Source: CAD feature listing. Evaluate the final solid. Frame: model axes, mm. Face numbers are marked on the shaded views. Give positions to 0.01 mm unless a question says otherwise; leave off trailing zeros. Order: outer loops, then holes, each group sorted by start corner. A loop starts at its lowest first (then second) coordinate and runs counter-clockwise, first axis right, second up. Notation, with made-up numbers: (9.5, 33.25) -> (22.5, 33.25) arc R35 ccw to (22.5, 69.25) -> close; hole circle Ø5 at (50.5, 68). An arc over 180 degrees is marked (long way). Use CSV: the item, a comma, the result in double quotes.
Autodesk Inventor part; units mm, degrees
ref_plane "YZ Plane" through (0, 0, 0) normal (1, 0, 0) x (0, 1, 0)
ref_plane "XZ Plane" through (0, 0, 0) normal (0, 1, 0) x (-1, 0, 0)
ref_plane "XY Plane" through (0, 0, 0) normal (0, 0, 1) x (1, 0, 0)
sketch "Sketch1" plane through (0, 0, 0) normal (0, 1, 0) x (-1, 0, 0)
  line L0 (6.29, 17.6429) -> (-24.19, 17.6429)
  line L1 (-24.19, 17.6429) -> (-24.19, -14.3571)
  line L2 (-24.19, -14.3571) -> (6.29, -14.3571)
  line L3 (6.29, -14.3571) -> (6.29, 17.6429)
  point P0 (0, 0)
  dimension "d0" = 30.48
  dimension "d1" = 32
extrude "Extrusion1" add sketch "Sketch1" along normal blind 2
sketch "Sketch3" plane through (0, 2, 0) normal (0, 1, 0) x (1, 0, 0)
  line L0 (-6.29, -17.6429) -> (24.19, -17.6429)
  line L1 (-6.29, -17.6429) -> (-6.29, -16.6429)
  line L2 (-6.29, 14.3571) -> (-6.29, -17.6429)
  line L3 (-6.29, -16.6429) -> (-5.29, -16.6429)
  line L4 (-5.29, -16.6429) -> (-5.29, 13.3571)
  line L5 (24.19, 14.3571) -> (-6.29, 14.3571)
  line L6 (24.19, -17.6429) -> (24.19, 14.3571)
  line L7 (24.19, -17.6429) -> (23.19, -17.6429)
  line L8 (23.19, -17.6429) -> (23.19, -16.6429)
  line L9 (23.19, -16.6429) -> (23.19, 3.3571)
  line L10 (23.19, -16.6429) -> (-5.29, -16.6429)
  line L11 (-5.29, -16.6429) -> (-5.29, 13.3571)
  line L12 (-5.29, 13.3571) -> (23.19, 13.3571)
  line L13 (23.19, 13.3571) -> (23.19, -16.6429)
  point P0 (0, 0)
  dimension "d4" = 1
  dimension "d5" = 1
  dimension "d6" = 30
  dimension "d7" = 1
extrude "Extrusion3" add sketch "Sketch3" along normal blind 1 contours L1 L3 L10 L8 L0 | L8 L9 L13 L12 L4 L3 L2 L5 L6 L0
sketch "Sketch4" plane through (0, 0, 0) normal (0, -1, 0) x (1, 0, 0)
  line L0 (24.19, -14.3571) -> (-6.29, -14.3571)
  line L1 (8.95, -14.3571) -> (8.95, -7.3571)
  point P0 (0, 0)
  dimension "d12" = 7
hole "Hole1" at (8.95, 0, -7.3571) direction (0, 1, 0) diameter 9 end through all
sketch "Sketch5" plane through (0, 3, 0) normal (0, 1, 0) x (1, 0, 0)
  line L0 (-6.29, -17.6429) -> (24.19, -17.6429)
  line L1 (8.95, -17.6429) -> (8.95, -0.6429)
  line L2 (8.95, -0.6429) -> (24.19, -0.6429)
  line L3 (24.19, -17.6429) -> (24.19, 14.3571)
  line L4 (24.19, -0.6429) -> (24.19, -4.1429)
  line L5 (24.19, -4.1429) -> (23.19, -4.1429)
  line L6 (23.19, -16.6429) -> (23.19, 13.3571)
  line L7 (23.19, -4.1429) -> (23.19, 2.8571)
  line L8 (23.19, 2.8571) -> (24.19, 2.8571)
  line L9 (24.19, 2.8571) -> (24.19, -4.1429)
  line L10 (-5.29, -16.6429) -> (-5.29, 13.3571)
  line L11 (-5.29, -0.6429) -> (-5.29, -4.1429)
  line L12 (-5.29, -4.1429) -> (-6.29, -4.1429)
  line L13 (-6.29, 14.3571) -> (-6.29, -17.6429)
  line L14 (-6.29, -4.1429) -> (-6.29, 2.8571)
  line L15 (-6.29, 2.8571) -> (-5.29, 2.8571)
  line L16 (-5.29, -0.6429) -> (-5.29, 2.8571)
  point P0 (0, 0)
  dimension "d20" = 17
  dimension "d21" = 3.5
  dimension "d22" = 7
  dimension "d23" = 7
sketch "Sketch6" plane through (0, 0, 0) normal (0, -1, 0) x (1, 0, 0)
  line L0 (-5.29, 4.1429) -> (-6.29, 4.1429)
  line L1 (-6.29, -2.8571) -> (-5.29, -2.8571)
  line L2 (23.19, -2.8571) -> (24.19, -2.8571)
  line L3 (24.19, 4.1429) -> (23.19, 4.1429)
  line L4 (-5.29, -13.3571) -> (-5.29, 16.6429)
  line L5 (-6.29, -14.3571) -> (-6.29, 17.6429)
  line L6 (23.19, 16.6429) -> (23.19, -13.3571)
  line L7 (24.19, 17.6429) -> (24.19, -14.3571)
  line L8 (24.19, 4.1429) -> (29.19, 4.1429)
  line L9 (29.19, 4.1429) -> (29.19, -2.8571)
  line L10 (29.19, -2.8571) -> (24.19, -2.8571)
  line L11 (-6.29, -2.8571) -> (-11.29, -2.8571)
  line L12 (-11.29, -2.8571) -> (-11.29, 4.1429)
  line L13 (-11.29, 4.1429) -> (-6.29, 4.1429)
  point P0 (0, 0)
  dimension "d26" = 5
  dimension "d27" = 5
extrude "Extrusion5" add sketch "Sketch6" against normal blind 3 contours L5 L11 L12 L13 | L7 L8 L9 L10
sketch "Sketch7" plane through (0, 0, 0) normal (0, -1, 0) x (1, 0, 0)
  line L0 (-6.29, 17.6429) -> (24.19, 17.6429)
  line L1 (8.95, 17.6429) -> (8.95, 0.6429)
  line L2 (8.95, 0.6429) -> (26.45, 0.6429)
  line L3 (26.45, 0.6429) -> (-8.55, 0.6429)
  point P0 (0, 0)
  dimension "d30" = 17
  dimension "d31" = 17.5
  dimension "d32" = 35
hole "Hole2" at (-8.55, 0, 0.6429) at (26.45, 0, 0.6429) direction (0, 1, 0) diameter 4 end through all
sketch "Sketch8" plane through (-6.29, 0, 17.6429) normal (0, 0, 1) x (1, 0, 0)
  line L0 (0, 0) -> (0, 3)
  line L1 (1, 3) -> (0, 3)
  line L2 (1, 3) -> (1, 3.5)
  line L3 (0, 3.5) -> (1, 3.5)
  line L4 (-5, 0) -> (-5, 3.25)
  line L5 (0, 0) -> (-5, 0)
  line L6 (0, 3) -> (0, 0)
  line L7 (0, 0) -> (30.48, 0)
  line L8 (30.48, 0) -> (30.48, 3)
  line L9 (0, 3) -> (30.48, 3)
  line L10 (0, 0) -> (0, 3)
  line L11 (0, 3.25) -> (0, 3.5)
  line L12 (-5, 3.25) -> (0, 3.25)
  point P0 (6.29, 0)
extrude "Extrusion6" cut sketch "Sketch8" against normal blind 0.2 contours L0 L1 L9 L8 L7
properties part number "sheel"
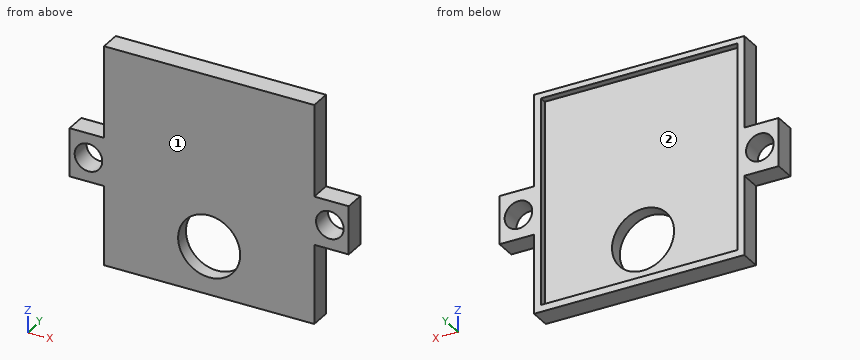
1. Mould query, pull axis Z, two halves, no side actions, for the marked faces 1 and 2. Classes: released by +Z, released by -Z, zero draft, split by the parting line, or undercut.
Answer below:
face 1,"zero draft"
face 2,"undercut"
2. Section query B-B on y = 2.45. Return loops of the section in (x, z), plus the area to 3 significant figures.
Answer below:
outline,"(-11.29, -2.86) -> (-6.29, -2.86) -> (-6.29, -14.36) -> (24.19, -14.36) -> (24.19, -2.86) -> (29.19, -2.86) -> (29.19, 4.14) -> (24.19, 4.14) -> (24.19, 17.44) -> (-6.29, 17.44) -> (-6.29, 4.14) -> (-11.29, 4.14) -> close; hole circle Ø4 at (-8.55, 0.64); hole (-5.29, -13.36) -> (23.19, -13.36) -> (23.19, 16.64) -> (-5.29, 16.64) -> close; hole circle Ø4 at (26.45, 0.64)"
area,"160 mm²"
3. Section query A-A on x = -8.55. Return loops of the section in (y, z).
Answer below:
outline,"(0, -2.86) -> (3, -2.86) -> (3, -1.36) -> (0, -1.36) -> close; (0, 2.64) -> (3, 2.64) -> (3, 4.14) -> (0, 4.14) -> close"
4. Ray query, line 1 along Z through (x, y) = (18, 2.9); line 2 along Z through (x, y) = (26.45, 1.3); line 3 along X through (y, z) = (2.45, -11). Return the intervals inside material, ascending.
Answer below:
line 1,"z = -14.36 to -13.36, 16.64 to 17.44"
line 2,"z = -2.86 to -1.36, 2.64 to 4.14"
line 3,"x = -6.29 to -5.29, 23.19 to 24.19"
5. Section query D-D on x = 3. Return loops of the section in (y, z), plus the area to 3 significant figures.
Answer below:
outline,"(0, -14.36) -> (3, -14.36) -> (3, -13.36) -> (2, -13.36) -> (2, 16.64) -> (3, 16.64) -> (3, 17.44) -> (0, 17.44) -> close"
area,"65.4 mm²"
6. Pin query (flat end, axial travel): P1, Ø1, axis at y = 2, z = -6, coming from the +X side; P2, Ø0.9, axis at x = 26.5, y = 1, coming from the -Z side; P3, Ø1.5, axis at x = 27.5, y = 1.5, coming from the +Z side. Return the tip coordinate at first contact, or that it passes through.
Answer below:
P1,"stops at x = 24.19"
P2,"stops at z = -2.86"
P3,"stops at z = 4.14"
7. Section query C-C on z = -8. Return loops of the section in (x, y).
Answer below:
outline,"(-6.29, 0) -> (4.5, 0) -> (4.5, 2) -> (-5.29, 2) -> (-5.29, 3) -> (-6.29, 3) -> close; (13.4, 0) -> (24.19, 0) -> (24.19, 3) -> (23.19, 3) -> (23.19, 2) -> (13.4, 2) -> close"
